Verification items for the finished model (mm, model axes). Face numbers are marked on the shaded views. A direction names the side the tool comes from. Give positions to 0.01 mm unless a question says otherwise; leave off trailing zeros. Loops run counter-clockwise (first coordinate to the right, second up) from the corner with the lowest first, then second, coordinate; pieces in that order, holes last. Notation, with made-up numbers: M 41.25,13 L 56.25,13 A22 cw 56.25,27 Z; hole C -38.75,-22 d5. An arc over 180 degrees is marked long. Use a Markdown table: item, result.
from build123d import *

# Parameters (mm, degrees)
SKETCH1_R           = 10.4521
BOSS_EXTRUDE1_DEPTH = 1.9
SKETCH2_R           = 4.41325
BOSS_EXTRUDE2_DEPTH = 3.556
SKETCH3_R           = 1.49225
SKETCH3_R_2         = 0.81915
CUT_EXTRUDE1_DEPTH  = 16.756291595
SKETCH4_R           = 2.9337
CUT_EXTRUDE2_DEPTH  = 3.556


with BuildPart() as part:
    # Sketch1 → Boss-Extrude1 (new body)
    with BuildSketch(Plane(origin=(0, 0, 0), x_dir=(1, 0, 0), z_dir=(0, 1, 0))):
        with Locations(Location((0, 0, 0), (0, 0, 90))):
            Circle(SKETCH1_R)
    extrude(amount=BOSS_EXTRUDE1_DEPTH)

    # Sketch2 → Boss-Extrude2 (add)
    with BuildSketch(Plane(origin=(0, 1.9, 0), x_dir=(1, 0, 0), z_dir=(0, 1, 0))):
        with Locations(Location((0, 0, 0), (0, 0, 270))):
            Circle(SKETCH2_R)
    extrude(amount=BOSS_EXTRUDE2_DEPTH)

    # Sketch3 → Cut-Extrude1 (cut, through all)
    with BuildSketch(Plane.XZ):
        with Locations(Location((0, 0, 0), (0, 0, 270))):
            Circle(SKETCH3_R)
        with Locations(Location((-7.5057, 0, 0), (0, 0, 270))):
            Circle(SKETCH3_R_2)
        with Locations(Location((-7.5057, 3.49885, 0), (0, 0, 270))):
            Circle(SKETCH3_R_2)
        with Locations(Location((-7.5057, -3.49885, 0), (0, 0, 270))):
            Circle(SKETCH3_R_2)
        with Locations(Location((0, 7.5057, 0), (0, 0, 270))):
            Circle(SKETCH3_R_2)
        with Locations(Location((3.49885, 7.5057, 0), (0, 0, 270))):
            Circle(SKETCH3_R_2)
        with Locations(Location((-3.49885, 7.5057, 0), (0, 0, 270))):
            Circle(SKETCH3_R_2)
        with Locations(Location((7.5057, 0, 0), (0, 0, 270))):
            Circle(SKETCH3_R_2)
        with Locations(Location((7.5057, -3.49885, 0), (0, 0, 270))):
            Circle(SKETCH3_R_2)
        with Locations(Location((7.5057, 3.49885, 0), (0, 0, 270))):
            Circle(SKETCH3_R_2)
        with Locations(Location((0, -7.5057, 0), (0, 0, 270))):
            Circle(SKETCH3_R_2)
        with Locations(Location((-3.49885, -7.5057, 0), (0, 0, 270))):
            Circle(SKETCH3_R_2)
        with Locations(Location((3.49885, -7.5057, 0), (0, 0, 270))):
            Circle(SKETCH3_R_2)
    extrude(amount=-CUT_EXTRUDE1_DEPTH, mode=Mode.SUBTRACT)

    # Sketch4 → Cut-Extrude2 (cut)
    with BuildSketch(Plane(origin=(0, 5.456, 0), x_dir=(1, 0, 0), z_dir=(0, 1, 0))):
        with Locations(Location((0, 0, 0), (0, 0, 270))):
            Circle(SKETCH4_R)
    extrude(amount=-CUT_EXTRUDE2_DEPTH, mode=Mode.SUBTRACT)


solid = part.part
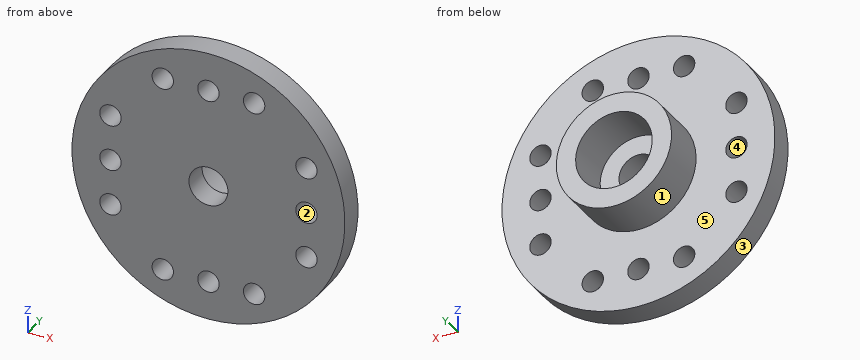
(1) Cross-section at A-A on z = 0. Record the cut outline in (x, y), then the cut area to 3 significant figures.
Results below:
| item | result |
|---|---|
| outline | M -10.45,0 L -8.32,0 L -8.32,1.9 L -10.45,1.9 Z; M -6.69,0 L -1.49,0 L -1.49,1.9 L -2.93,1.9 L -2.93,5.46 L -4.41,5.46 L -4.41,1.9 L -6.69,1.9 Z; M 1.49,0 L 6.69,0 L 6.69,1.9 L 4.41,1.9 L 4.41,5.46 L 2.93,5.46 L 2.93,1.9 L 1.49,1.9 Z; M 8.32,0 L 10.45,0 L 10.45,1.9 L 8.32,1.9 Z |
| area | 38.3 mm^2 |
(2) Draft check along Z on the marked faces 3, 4 and 5. Enter one of: +Z half, -Z half, draft (parallel to the pull), parting line (faces both ways), or undercut.
Results below:
| item | result |
|---|---|
| face 3 | parting line |
| face 4 | undercut |
| face 5 | draft |
(3) Cross-section at B-B on x = 0. Record the cut outline in (y, z), then the cut area to 3 significant figures.
Results below:
| item | result |
|---|---|
| outline | M 0,-10.45 L 1.9,-10.45 L 1.9,-8.32 L 0,-8.32 Z; M 0,-6.69 L 1.9,-6.69 L 1.9,-4.41 L 5.46,-4.41 L 5.46,-2.93 L 1.9,-2.93 L 1.9,-1.49 L 0,-1.49 Z; M 0,1.49 L 1.9,1.49 L 1.9,2.93 L 5.46,2.93 L 5.46,4.41 L 1.9,4.41 L 1.9,6.69 L 0,6.69 Z; M 0,8.32 L 1.9,8.32 L 1.9,10.45 L 0,10.45 Z |
| area | 38.3 mm^2 |
(4) Cross-section at D-D on y = 4.45. Record the cut outline in (x, z).
Results below:
| item | result |
|---|---|
| outline | C 0,0 d8.83; hole C 0,0 d5.87 |
(5) Gauge pin test, flat ends, axial feed: P1, Ø2, axis at x = -6, z = 2, coming from the +Y side; P2, Ø3, axis at x = 4, y = 1, coming from the +Z side. Record the tip position at first contact, or that the pin passes through.
Results below:
| item | result |
|---|---|
| P1 | y = 1.9 |
| P2 | z = 10.15 |
(6) Set-up check for the marked faces 1 and 2: record each of +Z, -Z, +X, -X, +Y, -Y from which the full face is reachable in a straight line by a thin tool's end or side.
Results below:
| item | result |
|---|---|
| face 1 | +Y |
| face 2 | +Y, -Y |
(7) Material ranges on line 1 (X direction, y = 1.2, z = 0); line 2 (Z direction, x = 7, y = 1.75); line 3 (X direction, y = 4.85, z = 2.5), recorded low to high.
Results below:
| item | result |
|---|---|
| line 1 | -10.45 to -8.32, -6.69 to -1.49, 1.49 to 6.69, 8.32 to 10.45 |
| line 2 | -7.76 to -4.14, -2.85 to -0.64, 0.64 to 2.85, 4.14 to 7.76 |
| line 3 | -3.64 to -1.54, 1.54 to 3.64 |
(8) Cross-section at C-C on z = -3.25. Record the cut outline in (x, y), then the cut area to 3 significant figures.
Results below:
| item | result |
|---|---|
| outline | M -9.93,0 L -8.29,0 L -8.29,1.9 L -9.93,1.9 Z; M -6.73,0 L 6.73,0 L 6.73,1.9 L 2.99,1.9 L 2.99,5.46 L -2.99,5.46 L -2.99,1.9 L -6.73,1.9 Z; M 8.29,0 L 9.93,0 L 9.93,1.9 L 8.29,1.9 Z |
| area | 53.1 mm^2 |
